Verification items for the finished model (mm, model axes). A direction names the side the tool comes from. Coordinates: 2 decimals unless noted, no trailing zeros. Write each loop counter-clockwise with the first axis right and the second up, starting at its lowest first coordinate (ties: lowest second). Pieces come first, ordered by that corner, then holes. Notation, with made-up numbers: (-8.5, 25) -> (17.5, 25) arc R18 ccw to (17.5, 54) -> close; hole circle Ø8 at (-14.5, 2). An arc over 180 degrees is marked (long way). Use CSV: the item, a comma, the result in double quotes.
```python
from build123d import *

# Parameters (mm, degrees)
BOSS_EXTRUDE1_DEPTH      = 914.4
BOSS_EXTRUDE1_DEPTH_BACK = 914.4
SKETCH2_W                = 1066.8
SKETCH2_H                = 38.1
CUT_EXTRUDE1_DEPTH       = 77.2


with BuildPart() as part:
    # Sketch1 → Boss-Extrude1 (new body, two sides)
    with BuildSketch(Plane(origin=(0, 0, 0), x_dir=(0, 0, -1), z_dir=(1, 0, 0))) as boss_extrude1_sk:
        with BuildLine():
            Line((0, 76.2), (0, 0))
            Line((0, 0), (76.2, 0))
            Line((76.2, 0), (76.2, 1.27))
            ThreePointArc((76.2, 1.27), (74.712102448, 4.862102448), (71.12, 6.35))
            Line((71.12, 6.35), (11.43, 6.35))
            ThreePointArc((11.43, 6.35), (7.837897552, 7.837897552), (6.35, 11.43))
            Line((6.35, 11.43), (6.35, 71.12))
            ThreePointArc((6.35, 71.12), (4.862102448, 74.712102448), (1.27, 76.2))
            Line((1.27, 76.2), (0, 76.2))
        make_face()
    extrude(amount=BOSS_EXTRUDE1_DEPTH)
    extrude(boss_extrude1_sk.sketch, amount=-BOSS_EXTRUDE1_DEPTH_BACK)

    # Sketch2 → Cut-Extrude1 (cut, through all)
    with BuildSketch(Plane.XY):
        with Locations((0, 57.15)):
            Rectangle(SKETCH2_W, SKETCH2_H)
    extrude(amount=-CUT_EXTRUDE1_DEPTH, mode=Mode.SUBTRACT)


solid = part.part
```
1) Gauge pin test, flat ends, axial feed: pin 1 (7 mm diameter, centred on x = 262.5, z = -3.5, fed in from +Y); pin 2 (1.5 mm diameter, centred on y = 9, z = -39.5, fed in from -X). Record the tip position at first contact, or that the pin passes through.
Return value:
pin 1,"y = 38.1"
pin 2,"through"
2) Set-up check for faces 1 (the flat face through (13, 0, -38)), 2 (the flat face through (13, 6.35, -42)): record each of +Z, -Z, +X, -X, +Y, -Y from which the full face is reachable in a straight line by a thin tool's end or side.
Return value:
face 1,"+Z, -Z, +X, -X, -Y"
face 2,"-Z, +X, -X, +Y"
3) Cross-section at B-B (z = -55). Record the boundary of the cut face in (x, y).
Return value:
outline,"(-914.4, 0) -> (914.4, 0) -> (914.4, 6.35) -> (-914.4, 6.35) -> close"
4) Cross-section at A-A (x = 791). Record the boundary of the cut face in (y, z), plus the area to 3 significant figures.
Return value:
outline,"(0, -76.2) -> (1.27, -76.2) arc R5.08 ccw to (6.35, -71.12) -> (6.35, -11.43) arc R5.08 cw to (11.43, -6.35) -> (71.12, -6.35) arc R5.08 ccw to (76.2, -1.27) -> (76.2, 0) -> (0, 0) -> close"
area,"922 mm2"
5) Scan lines: L1, parallel to Z at x = -785.5, y = 36; L2, parallel to Y at x = 302, z = -58.5; L3, parallel to Z at x = 588, y = 10. Record each from-to range of solid material in increasing order.
Return value:
L1,"-6.35 to 0"
L2,"0 to 6.35"
L3,"-6.56 to 0"
6) Cross-section at C-C (x = -515.5). Record the boundary of the cut face in (y, z), plus the area to 3 significant figures.
Return value:
outline,"(0, -76.2) -> (1.27, -76.2) arc R5.08 ccw to (6.35, -71.12) -> (6.35, -11.43) arc R5.08 cw to (11.43, -6.35) -> (38.1, -6.35) -> (38.1, 0) -> (0, 0) -> close"
area,"685 mm2"
